Design review of the part built by this model. Coordinates are the model's own, in mm. Coordinates: 2 decimals unless noted, no trailing zeros. Loops run counter-clockwise (first coordinate to the right, second up) from the corner with the lowest first, then second, coordinate; pieces in that order, holes last. Notation, with made-up numbers: (73, 19) - (110, 19) arc R12 cw to (110, 23) - close; hole circle Ø8 at (45.5, -38). An arc over 180 degrees is marked (long way). One line per question, with ' | ' between items.
from build123d import *

# Parameters (mm, degrees)
F0_W     = 60
F0_H     = 25
F1_DEPTH = 6
F3_D     = 5.8
F4_SIZE  = 5


with BuildPart() as f1:
    # F0 (on Top) → F1 (new body)
    with BuildSketch(Plane.XY):
        with Locations((30, 12.5)):
            Rectangle(F0_W, F0_H)
    extrude(amount=F1_DEPTH)

    # F3 (through all)
    with Locations(Plane.XY.offset(6)):
        with Locations((50, 7.5), (10, 7.5)):
            Hole(F3_D / 2)

    # F4
    f4_edges = [f1.edges().sort_by_distance(p)[0] for p in [
        (60, 25, 3),
        (0, 25, 3),
    ]]
    chamfer(f4_edges, length=F4_SIZE)


solid = f1.part
Q1. Take a section at D-D (x = 9). Give the boundary of the cut face in (y, z), plus the area to 3 significant figures.
Returned:
outline: (0, 0) - (4.78, 0) - (4.78, 6) - (0, 6) - close; (10.22, 0) - (25, 0) - (25, 6) - (10.22, 6) - close | area: 117 mm²
Q2. To check wall thickness, follow line 1 along Y through (x, z) = (10, 3.45); line 2 along X through (y, z) = (6.75, 1.45); line 3 along X through (y, z) = (7, 1.4). State the ranges of each line that lie inside material, in increasing order.
Returned:
line 1: y = 0 to 4.6, 10.4 to 25 | line 2: x = 0 to 7.2, 12.8 to 47.2, 52.8 to 60 | line 3: x = 0 to 7.14, 12.86 to 47.14, 52.86 to 60
Q3. Take a section at C-C (z = 2.9). Give the boundary of the cut face in (x, y), plus the area to 3 significant figures.
Returned:
outline: (0, 0) - (60, 0) - (60, 20) - (55, 25) - (5, 25) - (0, 20) - close; hole circle Ø5.8 at (10, 7.5); hole circle Ø5.8 at (50, 7.5) | area: 1,420 mm²
Q4. Take a section at A-A (x = 50). Give the boundary of the cut face in (y, z), plus the area to 3 significant figures.
Returned:
outline: (0, 0) - (4.6, 0) - (4.6, 6) - (0, 6) - close; (10.4, 0) - (25, 0) - (25, 6) - (10.4, 6) - close | area: 115 mm²
Q5. Draft analysis for pull direction X (two halves, no side actions). For faces 1 (the cylindrical face through (12.9, 7.6, 3)), 2 (the flat face through (30, 13, 0)), 3 (the flat face through (60, 10, 3)), 4 (the flat face through (0, 10, 3)), state which applies: +X half, -X half, draft (parallel to the pull), parting line (faces both ways), or undercut.
Returned:
face 1: undercut | face 2: draft | face 3: +X half | face 4: -X half
Q6. Take a section at B-B (y = 7.5). Give the boundary of the cut face in (x, z), plus the area to 3 significant figures.
Returned:
outline: (0, 0) - (7.1, 0) - (7.1, 6) - (0, 6) - close; (12.9, 0) - (47.1, 0) - (47.1, 6) - (12.9, 6) - close; (52.9, 0) - (60, 0) - (60, 6) - (52.9, 6) - close | area: 290 mm²
